from build123d import *

# Parameters (mm, degrees)
SKETCH_1_W      = 119.3
SKETCH_1_H      = 66
EXTRUDE_1_DEPTH = 2
SKETCH_2_W      = 78
SKETCH_2_H      = 5
EXTRUDE_2_DEPTH = 10.3
SKETCH_3_W      = 7
SKETCH_3_H      = 3
SKETCH_3_W_2    = 6
SKETCH_3_H_2    = 2
EXTRUDE_3_DEPTH = 10


with BuildPart() as part:
    # Эскиз1 → Бобышка-Вытянуть1 (new body)
    with BuildSketch(Plane(origin=(0, 0, 0), x_dir=(1, 0, 0), z_dir=(0, 1, 0))):
        with Locations((59.65, 33)):
            Rectangle(SKETCH_1_W, SKETCH_1_H)
    extrude(amount=EXTRUDE_1_DEPTH)

    # Эскиз2 → Бобышка-Вытянуть2 (add)
    with BuildSketch(Plane.XZ):
        with Locations((40, -9.5)):
            Rectangle(SKETCH_2_W, SKETCH_2_H)
        with Locations((40, -56.5)):
            Rectangle(SKETCH_2_W, SKETCH_2_H)
    extrude(amount=EXTRUDE_2_DEPTH)

    # Эскиз3 → Бобышка-Вытянуть3 (add)
    with BuildSketch(Plane.ZY):
        with Locations((-33, -1.5)):
            Rectangle(SKETCH_3_W, SKETCH_3_H)
        with Locations((-33, -1.5)):
            Rectangle(SKETCH_3_W_2, SKETCH_3_H_2, mode=Mode.SUBTRACT)
    extrude(amount=-EXTRUDE_3_DEPTH)


solid = part.part
Work out the finished part from the listing and answer in its coordinate system (mm). A direction names the side the tool comes from. Give positions to 0.01 mm unless a question says otherwise; leave off trailing zeros. Write each loop counter-clockwise with the first axis right and the second up, starting at its lowest first coordinate (ties: lowest second). Pieces come first, ordered by that corner, then holes. Notation, with made-up numbers: (11.25, 60) - (21.25, 60) arc R25 ccw to (21.25, 93) - close; hole circle Ø11 at (16, 39). An arc over 180 degrees is marked (long way). One line per item, written item: value. Start each with the question number.
1. Find section B-B (x = 7). Write down the section's boundary in (y, z), then the cut area to 3 significant figures.
2. Find section A-A (y = -5.5). Write down the section's boundary in (x, z).
3. Find section C-C (x = 65). Write down the section's boundary in (y, z).
4. For faces 1 (the flat face through (79, -5, -10)), 2 (the flat face through (1, -5, -10)), 3 (the flat face through (5, -3, -33)), determine the directions among +Z, -Z, +X, -X, +Y, -Y from which every point of the face is accessible in a straight line to the end or side of a thin tool.
5. Find section D-D (z = -14). Write down the section's boundary in (x, y).
6. Consider probe 1 along Y at (x, z) = (9.5, -32); probe 2 along Z at (x, y) = (72, -1.25); probe 3 along Y at (x, z) = (98.5, -56). Determine where each line is inside the solid, lowest interval first.
7. For a pull along Z with two mould halves and no side action, classify faces 4 (the flat face through (39, -5, -12)), 5 (the flat face through (5, -0.5, -33)), 6 (the flat face through (39, -10.3, -56)), 7 (the flat face through (39, -5, -59)) as +Z half, -Z half, draft (parallel to the pull), parting line (faces both ways), or undercut.
8. Given pin 1 (1.5 mm diameter, centred on x = 6.5, y = -2, fed in from -Z); pin 2 (0.6 mm diameter, centred on x = 3.5, y = -2, fed in from +Z); pin 3 (1.5 mm diameter, centred on y = -7, z = -10.5, fed in from -X); pin 4 (3 mm diameter, centred on y = -0.5, z = -24, fed in from +X), each flat-ended and moving along its own axis, determine where each tip first touches the part or whether it passes through.
Geometry results:
1. outline: (-10.3, -59) - (0, -59) - (0, -66) - (2, -66) - (2, 0) - (0, 0) - (0, -7) - (-10.3, -7) - (-10.3, -12) - (0, -12) - (0, -29.5) - (-3, -29.5) - (-3, -36.5) - (0, -36.5) - (0, -54) - (-10.3, -54) - close; hole (-2.5, -36) - (-0.5, -36) - (-0.5, -30) - (-2.5, -30) - close
1. area: 244 mm2
2. outline: (1, -59) - (79, -59) - (79, -54) - (1, -54) - close; (1, -12) - (79, -12) - (79, -7) - (1, -7) - close
3. outline: (-10.3, -59) - (0, -59) - (0, -66) - (2, -66) - (2, 0) - (0, 0) - (0, -7) - (-10.3, -7) - (-10.3, -12) - (0, -12) - (0, -54) - (-10.3, -54) - close
4. face 1: +Z, -Z, +X, -Y
4. face 2: +Z, -X, -Y
4. face 3: +X, -X, -Y
5. outline: (0, 0) - (119.3, 0) - (119.3, 2) - (0, 2) - close
6. probe 1: -3 to -2.5, -0.5 to 2
6. probe 2: -59 to -54, -12 to -7
6. probe 3: 0 to 2
7. face 4: undercut
7. face 5: undercut
7. face 6: draft
7. face 7: -Z half
8. pin 1: z = -59
8. pin 2: z = -7
8. pin 3: x = 1
8. pin 4: x = 119.3
